Build history of the part. All positions in model axes, mm. A direction names the side the tool comes from. Give positions to 0.01 mm unless a question says otherwise; leave off trailing zeros. Loops run counter-clockwise (first coordinate to the right, second up) from the corner with the lowest first, then second, coordinate; pieces in that order, holes last.
1) Band-saw the part on C-C on y = 14. List the corners of the cut face in (x, z) (3 decimals), then the cut area to 3 significant figures.
2) Band-saw the part on D-D on z = 33.5. State how many separate pieces and enclosed holes the cut face has, then the cut area to 3 significant figures.
3) Band-saw the part on A-A on y = 0. List the corners of the cut face in (x, z), then the cut area to 3 significant figures.
4) Flat gauge pins, fed straight in: P1, Ø10, axis at x = 17, z = 25.5, coming from the +Y side; P2, Ø6, axis at y = -3.5, z = 11.5, coming from the -X side; P3, Ø0.6, axis at y = 3.5, z = 12.5, coming from the +X side; P4, Ø12, axis at y = -3.5, z = 32, coming from the +X side. Where does each tip first touch, or does it go through?
5) Two-plate mould, pull along Y, no slides. Class faces 1 (the flat face through (19, 0, 7.057)), 2 (the flat face through (19, 0, 4.517)): +Y half, -Y half, draft (parallel to the pull), parting line (faces both ways), or undercut.
6) 3-axis set-ups, long thin cutter, end or side, ignore diameter. For faces 3 (the cylindrical face through (5.694, 10.046, 31.525)), 4 (the flat face through (25, -16, 55.317)): which of +Z, -Z, +X, -X, +Y, -Y reach the whole face in a straight line?
7) Wall check: line 1 (X direction, y = 0, z = 46); line 2 (X direction, y = 0, z = 33); line 3 (X direction, y = 0, z = 20). Give the ranges that are in metal, low to high.
8) Band-saw the part on B-B on x = 23. List the corners of the cut face in (y, z).
```python
from build123d import *

# Parameters (mm, degrees)
F0_W     = 19.05
F0_H     = 50.8
F2_T     = -2.54
F3_R     = 3.81
F4_ANGLE = 180


with BuildPart() as f1:
    # F0 (on Front) → F1 (revolve)
    with BuildSketch(Plane.XZ):
        with Locations((28.321, 29.9166932978)):
            Rectangle(F0_W, F0_H)
    revolve(axis=Axis((18.796, 0, 29.9166932978), (0, 0, -1)))

    # F2
    f2_openings = [f1.faces().sort_by_distance(p)[0] for p in [
        (18.796, 0, 55.316693),
    ]]
    offset(amount=F2_T, openings=f2_openings)

    # F3 (on Right) → F4 (revolve)
    with BuildSketch(Plane.YZ):
        with Locations((0, 13.575695168)):
            Circle(F3_R)
    revolve(axis=Axis((0, -0.5171763977, 27.0786721792), (0, 1, 0)), revolution_arc=F4_ANGLE)


solid = f1.part
```
Findings below:
1. outline: (5.877, 4.517) - (31.715, 4.517) - (31.715, 55.317) - (27.547, 55.317) - (27.547, 7.057) - (10.045, 7.057) - (10.045, 55.317) - (5.877, 55.317) - close
1. area: 468 mm2
2. separate pieces: 2
2. enclosed holes: 1
2. area: 336 mm2
3. outline: (-0.25, 4.52) - (37.85, 4.52) - (37.85, 55.32) - (35.31, 55.32) - (35.31, 7.06) - (2.29, 7.06) - (2.29, 55.32) - (-0.25, 55.32) - (-0.25, 44.39) arc R17.31 ccw to (-0.25, 9.77) - close; hole (-0.25, 17.39) - (-0.25, 36.77) arc R9.69 ccw to start
3. area: 661 mm2
4. P1: stops at y = 19.05
4. P2: stops at x = -10.61
4. P3: stops at x = 37.58
4. P4: stops at x = 37.85
5. face 1: undercut
5. face 2: draft
6. face 3: +Z
6. face 4: +Z, +X, -X, +Y, -Y
7. line 1: x = -0.25 to 2.29, 35.31 to 37.85
7. line 2: x = -16.27 to -7.67, -0.25 to 2.29, 35.31 to 37.85
7. line 3: x = -15.8 to -6.62, -0.25 to 2.29, 35.31 to 37.85
8. outline: (-18.58, 4.52) - (18.58, 4.52) - (18.58, 55.32) - (15.97, 55.32) - (15.97, 7.06) - (-15.97, 7.06) - (-15.97, 55.32) - (-18.58, 55.32) - close
